Autodesk Inventor part; units mm, degrees
ref_plane "YZ Plane" through (0, 0, 0) normal (1, 0, 0) x (0, 1, 0)
ref_plane "XZ Plane" through (0, 0, 0) normal (0, 1, 0) x (-1, 0, 0)
ref_plane "XY Plane" through (0, 0, 0) normal (0, 0, 1) x (1, 0, 0)
sketch "Sketch1" plane through (0, 0, 0) normal (0, 1, 0) x (-1, 0, 0)
  line L0 (533, 337) -> (-533, 337)
  line L1 (-533, 337) -> (-533, -337)
  line L2 (-533, -337) -> (533, -337)
  line L3 (533, -337) -> (533, 337)
  line L4 (533, 337) -> (-533, -337) construction
  line L5 (-533, 337) -> (533, -337) construction
  line L6 (531, 335) -> (-531, 335)
  line L7 (-531, 335) -> (-531, -335)
  line L8 (-531, -335) -> (531, -335)
  line L9 (531, -335) -> (531, 335)
  line L10 (531, 335) -> (-531, -335) construction
  line L11 (-531, 335) -> (531, -335) construction
  line L12 (503, 307) -> (-503, 307)
  line L13 (-503, 307) -> (-503, -307)
  line L14 (-503, -307) -> (503, -307)
  line L15 (503, -307) -> (503, 307)
  line L16 (503, 307) -> (-503, -307) construction
  line L17 (-503, 307) -> (503, -307) construction
  point P0 (0, 0)
  dimension "d0" = 1066
  dimension "d1" = 674
  dimension "d2" = 1062
  dimension "d3" = 670
  dimension "d4" = 1006
  dimension "d5" = 614
extrude "Extrusion1" add sketch "Sketch1" along normal blind 2 contours L9 L8 L7 L6
extrude "Extrusion2" add sketch "Sketch1" along normal blind 33 contours L3 L2 L1 L0
sketch "Sketch2" plane through (0, 33, 0) normal (0, 1, 0) x (1, 0, 0)
  line L0 (-533, -337) -> (533, -337)
  line L1 (533, -337) -> (533, 337)
  line L2 (533, 337) -> (-533, 337)
  line L3 (-533, 337) -> (-533, -337)
  line L4 (-533, -337) -> (533, 337) construction
  line L5 (533, -337) -> (-533, 337) construction
  line L6 (-523, -327) -> (523, -327)
  line L7 (523, -327) -> (523, 327)
  line L8 (523, 327) -> (-523, 327)
  line L9 (-523, 327) -> (-523, -327)
  line L10 (-523, -327) -> (523, 327) construction
  line L11 (523, -327) -> (-523, 327) construction
  point P0 (0, 0)
  dimension "d10" = 1066
  dimension "d11" = 674
  dimension "d12" = 1046
  dimension "d13" = 654
extrude "Extrusion3" add sketch "Sketch2" along normal blind 2
properties part number "frame"
Input: part model. Units: mm. Frame: model coordinates. A direction names the side the tool comes from. Give positions to 0.01 mm unless a question says otherwise; leave off trailing zeros. Order: outer loops, then holes, each group sorted by start corner. A loop starts at its lowest first (then second) coordinate and runs counter-clockwise, first axis right, second up. Notation, with made-up numbers: M -39.75,-28.75 L 3.25,-28.75 A20 ccw 3.25,-13.75 Z; hole C -29.75,40 d7. An arc over 180 degrees is marked long. Return JSON: item names as keys, results as strings.
Item 1: Access query for faces 1 (the flat face through (531, 17, 5)), 2 (the flat face through (-7, 17, 337)). Directions: +Z, -Z, +X, -X, +Y, -Y. A direction counts if a zero-diameter tool reaches every point of the face in a straight line with its end or side. Return the directions, or none.
Solutions:
{"face 1": "none", "face 2": "+Z, +X, -X, +Y, -Y"}
Item 2: Cut plane B-B (x = 441.5). Return loops of the section in (y, z).
Solutions:
{"outline": "M 0,-337 L 35,-337 L 35,-327 L 33,-327 L 33,-335 L 2,-335 L 2,-307 L 0,-307 Z; M 0,307 L 2,307 L 2,335 L 33,335 L 33,327 L 35,327 L 35,337 L 0,337 Z"}
Item 3: Cut plane C-C (z = -94.5). Return loops of the section in (x, y), then the cut area to 3 significant figures.
Solutions:
{"outline": "M -533,0 L -503,0 L -503,2 L -531,2 L -531,33 L -523,33 L -523,35 L -533,35 Z; M 503,0 L 533,0 L 533,35 L 523,35 L 523,33 L 531,33 L 531,2 L 503,2 Z", "area": "284 mm^2"}
Item 4: Pull-direction query (X, two-part tool) for faces 3 (the flat face through (-531, 17, -5)), 4 (the flat face through (-533, 17, -5)), 5 (the flat face through (42, 0, -323)); classes: +X half, -X half, draft (parallel to the pull), parting line (faces both ways), or undercut.
Solutions:
{"face 3": "undercut", "face 4": "-X half", "face 5": "draft"}
Item 5: Cut plane A-A (y = 22.5). Return loops of the section in (x, z).
Solutions:
{"outline": "M -533,-337 L 533,-337 L 533,337 L -533,337 Z; hole M -531,-335 L 531,-335 L 531,335 L -531,335 Z"}
Item 6: Ray query, probe 1 along Z at (x, y) = (372.5, 27); probe 2 along X at (y, z) = (24.5, -133.5); probe 3 along X at (y, z) = (33.5, 136.5). Return the intervals inside material, ascending.
Solutions:
{"probe 1": "-337 to -335, 335 to 337", "probe 2": "-533 to -531, 531 to 533", "probe 3": "-533 to -523, 523 to 533"}
